Read the model definition and answer for the solid it produces. Units are mm, in the model's axes. Round coordinates to 2 decimals unless told otherwise and drop trailing zeros. Order: outer loops, then holes, each group sorted by start corner. A loop starts at its lowest first (then second) coordinate and runs counter-clockwise, first axis right, second up. Notation, with made-up numbers: M 2.25,20.5 L 40.25,20.5 A25 ccw 40.25,45.5 Z; hole C -8,-17.5 d10. An arc over 180 degrees is marked long. Answer as CSV lines item,"result".
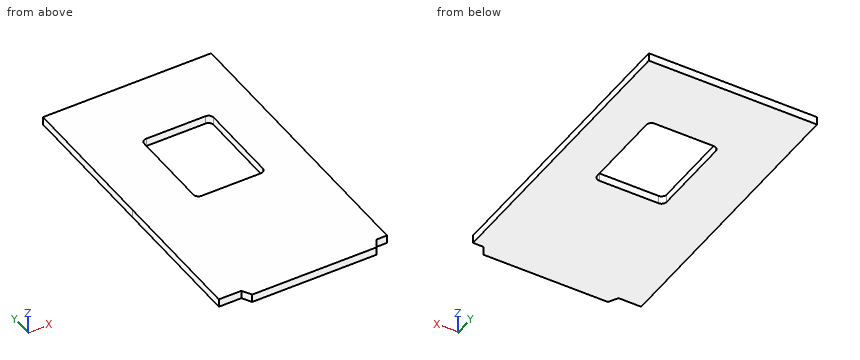
```python
from build123d import *
from OCP.BRepAlgoAPI import BRepAlgoAPI_Cut
from OCP.TopTools import TopTools_ListOfShape

# Parameters (mm, degrees)
SKETCH1_W           = 20
SKETCH1_H           = 30
BOSS_EXTRUDE1_DEPTH = 1.6
SKETCH2_W           = 1.6
SKETCH2_H           = 30
BOSS_EXTRUDE2_DEPTH = 13.22962
SKETCH3_W           = 33.229619685
SKETCH3_H           = 1.6
BOSS_EXTRUDE3_DEPTH = 29.21
CUT_EXTRUDE1_DEPTH  = 1.6
CUT_EXTRUDE2_DEPTH  = 29.21


with BuildPart() as part:
    # Sketch1 → Boss-Extrude1 (new body)
    with BuildSketch(Plane.XY):
        Rectangle(SKETCH1_W, SKETCH1_H)
    extrude(amount=BOSS_EXTRUDE1_DEPTH)

    # Sketch2 → Boss-Extrude2 (add)
    with BuildSketch(Plane.ZY.offset(10)):
        with Locations((0.8, 0)):
            Rectangle(SKETCH2_W, SKETCH2_H)
    extrude(amount=BOSS_EXTRUDE2_DEPTH)

    # Sketch3 → Boss-Extrude3 (add)
    with BuildSketch(Plane(origin=(0, 15, 0), x_dir=(1, 0, 0), z_dir=(0, 1, 0))):
        with Locations((-6.614809843, -0.8)):
            Rectangle(SKETCH3_W, SKETCH3_H)
    extrude(amount=BOSS_EXTRUDE3_DEPTH)

    # Sketch4 → Cut-Extrude1 (cut)
    with BuildSketch(Plane(origin=(0, 0, 0), x_dir=(-1, 0, 0), z_dir=(0, 0, -1))):
        with BuildLine():
            Line((-1.398817815, 13.19), (-1.398817815, 29.2))
            ThreePointArc((-1.398817815, 29.2), (-1.105924597, 29.907106781), (-0.398817815, 30.2))
            Line((-0.398817815, 30.2), (11.298057185, 30.2))
            ThreePointArc((11.298057185, 30.2), (12.005163966, 29.907106781), (12.298057185, 29.2))
            Line((12.298057185, 29.2), (12.298057185, 13.19))
            ThreePointArc((12.298057185, 13.19), (12.005163966, 12.482893219), (11.298057185, 12.19))
            Line((11.298057185, 12.19), (-0.398817815, 12.19))
            ThreePointArc((-0.398817815, 12.19), (-1.105924597, 12.482893219), (-1.398817815, 13.19))
        make_face()
    extrude(amount=-CUT_EXTRUDE1_DEPTH, mode=Mode.SUBTRACT)


with BuildPart() as cut_extrude2_tool:
    # Sketch5 → Cut-Extrude2 (new body)
    with BuildSketch(Plane(origin=(0, 0, 0), x_dir=(-1, 0, 0), z_dir=(0, 0, -1))):
        Polygon((-7.883969717, -13.186759938), (-6.837095086, -15), (-10, -15), (-10, -13.186759938), align=None)
        Polygon((17.736334458, -15), (18.783209096, -13.186759938), (19.63963747, -13.186759938), (23.229619685, -13.186759938), (23.229619685, -15), align=None)
    extrude(amount=-CUT_EXTRUDE2_DEPTH)


with BuildPart() as part_1:
    add(part.part)

    # Cut-Extrude2: cut by cut_extrude2_tool, with a tolerance
    cut_extrude2_stock = TopTools_ListOfShape()
    cut_extrude2_stock.Append(part_1.part.wrapped)
    cut_extrude2_tools = TopTools_ListOfShape()
    cut_extrude2_tools.Append(cut_extrude2_tool.part.wrapped)
    cut_extrude2_cut = BRepAlgoAPI_Cut()
    cut_extrude2_cut.SetArguments(cut_extrude2_stock)
    cut_extrude2_cut.SetTools(cut_extrude2_tools)
    cut_extrude2_cut.SetFuzzyValue(0.00001)
    cut_extrude2_cut.Build()
    add(Compound.cast(cut_extrude2_cut.Shape()).solids(), mode=Mode.REPLACE)


solid = part_1.part
```
Item 1: A cutting plane is placed at A-A, the plane x = -6. Determine the outline of the cut face in (y, z).
Ans:
outline,"M -15,0 L 12.19,0 L 12.19,1.6 L -15,1.6 Z; M 30.2,0 L 44.21,0 L 44.21,1.6 L 30.2,1.6 Z"
Item 2: Flat-ended cylindrical pins translate along their axes: pin 1 (12 mm diameter, centred on x = -6.5, y = 28, fed in from -Z); pin 2 (0.5 mm diameter, centred on x = 9, z = 1, fed in from -Y). Find the tip coordinate at first contact, or state that the pin passes through.
Ans:
pin 1,"z = 0"
pin 2,"y = -13.19"
Item 3: A cutting plane is placed at B-B, the plane y = 17. Determine the outline of the cut face in (x, z).
Ans:
outline,"M -23.23,0 L -12.3,0 L -12.3,1.6 L -23.23,1.6 Z; M 1.4,0 L 10,0 L 10,1.6 L 1.4,1.6 Z"
Item 4: Find the intervals of material crossed by probe 1 along Y at (x, z) = (-7.5, 1.15); probe 2 along X at (y, z) = (17.5, 0.2); probe 3 along Y at (x, z) = (1, 0.95), in increasing order. Write a range as [from, to].
Ans:
probe 1,"[-15, 12.19], [30.2, 44.21]"
probe 2,"[-23.23, -12.3], [1.4, 10]"
probe 3,"[-15, 12.39], [30, 44.21]"
Item 5: A cutting plane is placed at C-C, the plane z = 0.35. Determine the outline of the cut face in (x, y), and give its area (3 significant figures).
Ans:
outline,"M -23.23,-13.19 L -18.78,-13.19 L -17.74,-15 L 6.84,-15 L 7.88,-13.19 L 10,-13.19 L 10,44.21 L -23.23,44.21 Z; hole M -12.3,13.19 A1 ccw -11.3,12.19 L 0.4,12.19 A1 ccw 1.4,13.19 L 1.4,29.2 A1 ccw 0.4,30.2 L -11.3,30.2 A1 ccw -12.3,29.2 Z"
area,"1,710 mm2"
